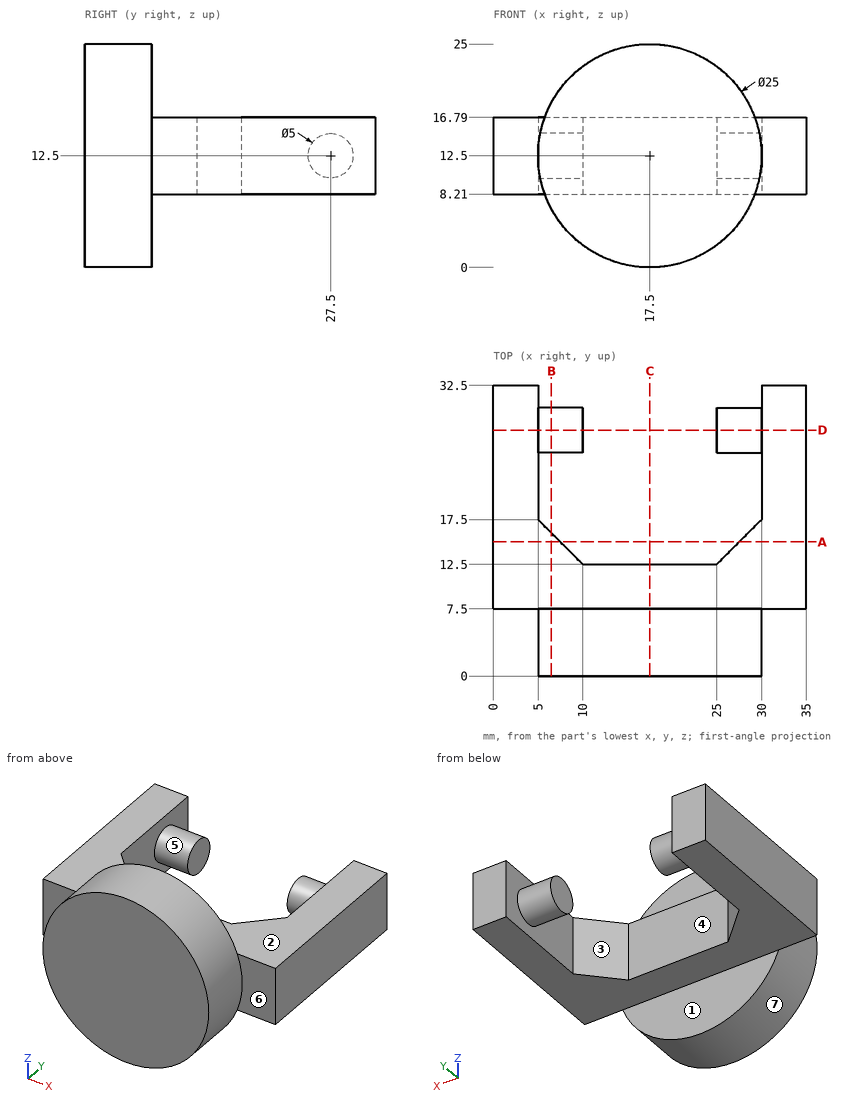
Geometry: see drawing. Coordinates: mm, zero at the bounding-box minimum. A direction names the side the tool comes from. Give positions to 0.01 mm unless a question says otherwise; leave off trailing zeros. Loops run counter-clockwise (first coordinate to the right, second up) from the corner with the lowest first, then second, coordinate; pieces in that order, holes last. Notation, with made-up numbers: (66.5, 49) -> (98.5, 49) arc R13 cw to (98.5, 57) -> close; hole circle Ø3 at (89, -16.5). An arc over 180 degrees is marked (long way). Use one line per item in the form item = value.
Item 1: Line query: probe 1 along Z at (x, y) = (7, 10.5); probe 2 along Y at (x, z) = (11.5, 17.5); probe 3 along X at (y, z) = (15, 10.75). Output: solid intervals per line, ascending.
A:
probe_1 = 8.21 to 16.79
probe_2 = 0 to 7.5
probe_3 = 0 to 7.5, 27.5 to 35
Item 2: Section query A-A on y = 15. Output: boundary loops of the cut face in (x, z).
A:
outline = (0, 8.21) -> (7.5, 8.21) -> (7.5, 16.79) -> (0, 16.79) -> close; (27.5, 8.21) -> (35, 8.21) -> (35, 16.79) -> (27.5, 16.79) -> close
Item 3: Pin query (flat end, axial travel): P1, Ø5, axis at x = 25, y = 6, coming from the +Z side; P2, Ø2, axis at x = 28, y = 7, coming from the -Z side (1 decimal); P3, Ø3, axis at x = 15.5, z = 7.5, coming from the +Y side; P4, Ø2.5, axis at y = 28, z = 12, coming from the -X side. Return the tip coordinate at first contact, or that it passes through.
A:
P1 = 23.96
P2 = 4.4
P3 = 12.5
P4 = 0
Item 4: Section query C-C on x = 17.5. Output: boundary loops of the cut face in (y, z).
A:
outline = (0, 0) -> (7.5, 0) -> (7.5, 8.21) -> (12.5, 8.21) -> (12.5, 16.79) -> (7.5, 16.79) -> (7.5, 25) -> (0, 25) -> close
Item 5: Draft query along X for the marked faces 5, 6 and 7. Return one class per face: pulls with the +X half, pulls with the -X half, needs draft (parallel to the pull), parting line crosses it, or undercut.
A:
face_5 = undercut
face_6 = needs draft
face_7 = parting line crosses it
Item 6: Section query D-D on y = 27.5. Output: boundary loops of the cut face in (x, z).
A:
outline = (0, 8.21) -> (5, 8.21) -> (5, 10) -> (10, 10) -> (10, 15) -> (5, 15) -> (5, 16.79) -> (0, 16.79) -> close; (25, 10) -> (30, 10) -> (30, 8.21) -> (35, 8.21) -> (35, 16.79) -> (30, 16.79) -> (30, 15) -> (25, 15) -> close
Item 7: Access query for the marked faces 1, 2, 3 and 4. Directions: +Z, -Z, +X, -X, +Y, -Y. A direction counts if a zero-diameter tool reaches every point of the face in a straight line with its end or side. Return the directions, or none.
A:
face_1 = -Z, +X, -X, +Y
face_2 = +Z, +X, -X, +Y
face_3 = +Z, -Z
face_4 = +Z, -Z, +Y
Item 8: Section query B-B on x = 6.5. Output: boundary loops of the cut face in (y, z).
A:
outline = (0, 6.56) -> (7.5, 6.56) -> (7.5, 8.21) -> (16, 8.21) -> (16, 16.79) -> (7.5, 16.79) -> (7.5, 18.44) -> (0, 18.44) -> close; circle Ø5 at (27.5, 12.5)
